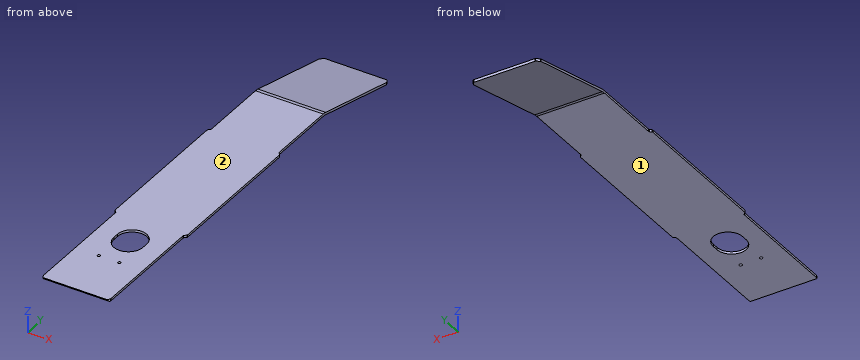
from build123d import *

# Parameters (mm, degrees)
SKETCH1_R              = 5
EXTRUDE1_DEPTH         = 8
PROCESS_BENDS1_START   = -116
PROCESS_BENDS1_DEPTH   = 232
PROCESS_BENDS1_2_DEPTH = 232
PROCESS_BENDS1_START_2 = 273
PROCESS_BENDS1_3_DEPTH = 10
SK_RPNING1_SIZE        = 6


with BuildPart() as part:
    # Sketch1 → Extrude1 (new body)
    with BuildSketch(Plane.XY):
        with BuildLine():
            Line((-108.645898034, 0), (108.645898034, 0))
            ThreePointArc((108.645898034, 0), (110.22309137, 0.448047575), (111.329179607, 1.658359214))
            Line((111.329179607, 1.658359214), (115.183281573, 9.366563146))
            ThreePointArc((115.183281573, 9.366563146), (115.419746968, 10.018945171), (115.5, 10.708203932))
            Line((115.5, 10.708203932), (115.5, 404.257359313))
            ThreePointArc((115.5, 404.257359313), (115.728361402, 405.40540961), (116.378679656, 406.378679656))
            Line((116.378679656, 406.378679656), (123.121320344, 413.121320344))
            ThreePointArc((123.121320344, 413.121320344), (123.771638598, 414.09459039), (124, 415.242640687))
            Line((124, 415.242640687), (124, 915.757359313))
            ThreePointArc((124, 915.757359313), (123.771638598, 916.90540961), (123.121320344, 917.878679656))
            Line((123.121320344, 917.878679656), (116.878679656, 924.121320344))
            ThreePointArc((116.878679656, 924.121320344), (116.228361402, 925.09459039), (116, 926.242640687))
            Line((116, 926.242640687), (116, 1522.091673087))
            ThreePointArc((116, 1522.091673087), (115.871276079, 1522.961025533), (115.496150883, 1523.755773675))
            Line((115.496150883, 1523.755773675), (106.890599608, 1536.664100589))
            ThreePointArc((106.890599608, 1536.664100589), (105.810022501, 1537.645023796), (104.394448725, 1538))
            Line((104.394448725, 1538), (-104.394448725, 1538))
            ThreePointArc((-104.394448725, 1538), (-105.810022501, 1537.645023796), (-106.890599608, 1536.664100589))
            Line((-106.890599608, 1536.664100589), (-115.496150883, 1523.755773675))
            ThreePointArc((-115.496150883, 1523.755773675), (-115.871276079, 1522.961025533), (-116, 1522.091673087))
            Line((-116, 1522.091673087), (-116, 926.242640687))
            ThreePointArc((-116, 926.242640687), (-116.228361402, 925.09459039), (-116.878679656, 924.121320344))
            Line((-116.878679656, 924.121320344), (-123.121320344, 917.878679656))
            ThreePointArc((-123.121320344, 917.878679656), (-123.771638598, 916.90540961), (-124, 915.757359313))
            Line((-124, 915.757359313), (-124, 415.242640687))
            ThreePointArc((-124, 415.242640687), (-123.771638598, 414.09459039), (-123.121320344, 413.121320344))
            Line((-123.121320344, 413.121320344), (-116.378679656, 406.378679656))
            ThreePointArc((-116.378679656, 406.378679656), (-115.728361402, 405.40540961), (-115.5, 404.257359313))
            Line((-115.5, 404.257359313), (-115.5, 10.708203932))
            ThreePointArc((-115.5, 10.708203932), (-115.419746968, 10.018945171), (-115.183281573, 9.366563146))
            Line((-115.183281573, 9.366563146), (-111.329179607, 1.658359214))
            ThreePointArc((-111.329179607, 1.658359214), (-110.22309137, 0.448047575), (-108.645898034, 0))
        make_face()
        with Locations((-35, 185)):
            Circle(SKETCH1_R, mode=Mode.SUBTRACT)
        with Locations(Location((35, 185, 0), (0, 0, 180))):
            Circle(SKETCH1_R, mode=Mode.SUBTRACT)
        with BuildLine():
            Line((-50, 290), (-50, 310))
            ThreePointArc((-50, 310), (0, 360), (50, 310))
            Line((50, 310), (50, 290))
            ThreePointArc((50, 290), (0, 240), (-50, 290))
        make_face(mode=Mode.SUBTRACT)
    extrude(amount=EXTRUDE1_DEPTH)

    # Process-Bends1: read off the stored shape, not the designer's step
    # Process-Bends1 outline → Process-Bends1 (cut)
    with BuildSketch(Plane.YZ.offset(PROCESS_BENDS1_START)):
        with BuildLine():
            Line((1180.17810598, 6.397455383), (1206.825425416, 0))
            Line((1206.825425416, 0), (1538, 0))
            Line((1538, 0), (1538, 8))
            Line((1538, 8), (1166.638274876, 8))
            ThreePointArc((1166.638274876, 8), (1173.455443929, 7.597970503), (1180.17810598, 6.397455383))
        make_face()
    extrude(amount=PROCESS_BENDS1_DEPTH, mode=Mode.SUBTRACT)

    # Process-Bends1 2 outline → Process-Bends1 2 (add)
    with BuildSketch(Plane.YZ.offset(PROCESS_BENDS1_START)):
        with BuildLine():
            Line((1527.039613862, -85.103946551), (1528.907176773, -77.324987188))
            Line((1528.907176773, -77.324987188), (1206.825425416, 0))
            Line((1206.825425416, 0), (1166.638274876, 0))
            ThreePointArc((1166.638274876, 0), (1172.515144749, -0.346577152), (1178.310543069, -1.38150398))
            Line((1178.310543069, -1.38150398), (1527.039613862, -85.103946551))
        make_face()
    extrude(amount=PROCESS_BENDS1_2_DEPTH)

    # Process-Bends1 3 outline → Process-Bends1 3 (cut)
    with BuildSketch(Plane(origin=(0, 0, 0), x_dir=(1, 0, 0), z_dir=(0, 0.2334453638559061, 0.9723699203976764)).offset(PROCESS_BENDS1_START_2)):
        with BuildLine():
            ThreePointArc((-116, 1488.806182631), (-115.871276079, 1489.675535077), (-115.496150883, 1490.470283219))
            Line((-115.496150883, 1490.470283219), (-106.890599608, 1503.378610132))
            ThreePointArc((-106.890599608, 1503.378610132), (-105.810022502, 1504.35953334), (-104.394448725, 1504.714509544))
            Line((-104.394448725, 1504.714509544), (-116, 1504.714509543))
            Line((-116, 1504.714509543), (-116, 1488.806182631))
        make_face()
        with BuildLine():
            Line((116, 1504.714509543), (104.394448725, 1504.714509544))
            ThreePointArc((104.394448725, 1504.714509544), (105.810022502, 1504.35953334), (106.890599608, 1503.378610132))
            Line((106.890599608, 1503.378610132), (115.496150883, 1490.470283219))
            ThreePointArc((115.496150883, 1490.470283219), (115.871276079, 1489.675535077), (116, 1488.806182631))
            Line((116, 1488.806182631), (116, 1504.714509543))
        make_face()
    extrude(amount=PROCESS_BENDS1_3_DEPTH, mode=Mode.SUBTRACT)

    # Skærpning1
    # the kernel refuses this chamfer: 6 mm, written as the material it takes off along each edge
    with BuildSketch(Plane(origin=(-124.075995962, 0, 0), x_dir=(0, 1, 0), z_dir=(1, 0, 0))) as sk_rpning1_piece_1:
        Polygon((SK_RPNING1_SIZE, 0), (0, SK_RPNING1_SIZE), (0, 0), align=None)
    extrude(amount=248.151991923, mode=Mode.SUBTRACT)
    with BuildSketch(Plane(origin=(-108.645898034, 3, 0), x_dir=(0.03163904554191759, -0.9994993600784327, 0), z_dir=(-0.9994993600784327, -0.03163904554191759, 0))) as sk_rpning1_piece_2_section:
        Polygon((0, 3), (3, SK_RPNING1_SIZE), (3, 0), (0, 0), align=None)
    sk_rpning1_piece_2 = revolve(axis=Axis((-108.645898034, 3, 0), (0, 0, 1)), revolution_arc=358.186913645, mode=Mode.PRIVATE)
    sk_rpning1_piece_2 = split(sk_rpning1_piece_2, bisect_by=Plane(origin=(-108.645898034, 4.5, 1.5), z_dir=(0, -0.7071067811865483, -0.7071067811865468)), keep=Keep.TOP, mode=Mode.PRIVATE)
    add(sk_rpning1_piece_2, mode=Mode.SUBTRACT)
    with BuildSketch(Plane(origin=(108.645898034, 3, 0), x_dir=(0, -1, 0), z_dir=(-1, 0, 0))) as sk_rpning1_piece_3_section:
        Polygon((0, 3), (3, SK_RPNING1_SIZE), (3, 0), (0, 0), align=None)
    sk_rpning1_piece_3 = revolve(axis=Axis((108.645898034, 3, 0), (0, 0, 1)), revolution_arc=358.186913645, mode=Mode.PRIVATE)
    sk_rpning1_piece_3 = split(sk_rpning1_piece_3, bisect_by=Plane(origin=(108.645898034, 4.5, 1.5), z_dir=(0, -0.7071067811865483, -0.7071067811865468)), keep=Keep.TOP, mode=Mode.PRIVATE)
    add(sk_rpning1_piece_3, mode=Mode.SUBTRACT)


solid = part.part
Geometry check sheet. Reference: the model listing, model coordinates, mm. Face numbers are marked on the shaded views. A direction names the side the tool comes from. Give positions to 0.01 mm unless a question says otherwise; leave off trailing zeros. Loops run counter-clockwise (first coordinate to the right, second up) from the corner with the lowest first, then second, coordinate; pieces in that order, holes last.
(1) Depth check by flat-ended pin: pin 1 Ø2.5 at (y, z) = (297.5, 5) entering from -X; pin 2 Ø9 at (y, z) = (301, 4.5) entering from +X; pin 3 Ø6 at (x, y) = (35, 185) entering from +Z; pin 4 Ø13 at (x, y) = (-35, 185) entering from +Z. Enter the tip coordinate at first touch or a pass-through.
From the geometry:
pin 1: stops at x = -115.5
pin 2: stops at x = 115.5
pin 3: passes through
pin 4: stops at z = 8
(2) Thickness scan on L1, parallel to Z at x = 6.5, y = 92; L2, parallel to Z at x = 91.5, y = 1243.5. Record the ranges inside material, lowest first.
From the geometry:
L1: z = 0 to 8
L2: z = -17.03 to -8.8
(3) Section check B-B on x = -81.5. Record the cut outline in (y, z).
From the geometry:
outline: (0, 6) - (6, 0) - (1166.64, 0) arc R50 cw to (1178.31, -1.38) - (1527.04, -85.1) - (1528.91, -77.32) - (1180.18, 6.4) arc R58 ccw to (1166.64, 8) - (0, 8) - close
(4) Set-up check for the marked faces 1 and 2: record each of +Z, -Z, +X, -X, +Y, -Y from which the full face is reachable in a straight line by a thin tool's end or side.
From the geometry:
face 1: -Z, +X, -X, -Y
face 2: +Z, +X, -X, +Y, -Y
(5) Section check C-C on y = 204. Record the cut outline in (x, z), then the cut area to 3 significant figures.
From the geometry:
outline: (-115.5, 0) - (115.5, 0) - (115.5, 8) - (-115.5, 8) - close
area: 1,850 mm2
(6) Section check A-A on x = 0. Record the cut outline in (y, z).
From the geometry:
outline: (0, 6) - (6, 0) - (240, 0) - (240, 8) - (0, 8) - close; (360, 0) - (1166.64, 0) arc R50 cw to (1178.31, -1.38) - (1527.04, -85.1) - (1528.91, -77.32) - (1180.18, 6.4) arc R58 ccw to (1166.64, 8) - (360, 8) - close
(7) Section check D-D on z = -31. Record the cut outline in (x, y).
From the geometry:
outline: (-116, 1301.68) - (116, 1301.68) - (116, 1335.95) - (-116, 1335.95) - close
